Model file for the job. Use its own axes, mm. Face numbers are marked on the shaded views. A direction names the side the tool comes from. Coordinates: 2 decimals unless noted, no trailing zeros. Write each loop counter-clockwise with the first axis right and the second up, starting at its lowest first coordinate (ties: lowest second). Pieces come first, ordered by that corner, then holes. Notation, with made-up numbers: (76, 58.25) -> (98, 58.25) arc R31 ccw to (98, 85.25) -> close; hole circle Ø10 at (-12, 41). An arc over 180 degrees is marked (long way). Answer as a JSON object with one key per item and string values. Group by question number.
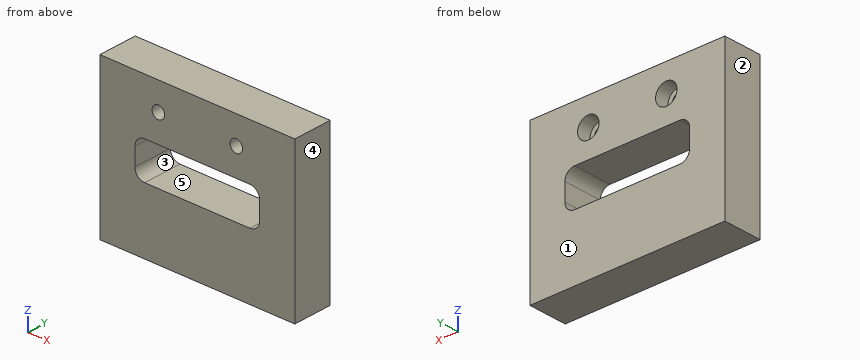
from build123d import *

# Parameters (mm, degrees)
SKETCH_1_W                = 100
SKETCH_1_H                = 80
SKETCH_1_W_2              = 64
SKETCH_1_H_2              = 19
EXTRUDE_1_DEPTH           = 20
FILLET_1_R                = 5
HOLE_WIZARD_1_D           = 6.4
HOLE_WIZARD_1_DEPTH       = 100
HOLE_WIZARD_1_CBORE_D     = 11
HOLE_WIZARD_1_CBORE_DEPTH = 7


with BuildPart() as part:
    # 草图1 → 凸台-拉伸1 (new body)
    with BuildSketch(Plane(origin=(0, 0, 0), x_dir=(1, 0, 0), z_dir=(0, 1, 0))):
        Rectangle(SKETCH_1_W, SKETCH_1_H)
        with Locations((0, -2.5)):
            Rectangle(SKETCH_1_W_2, SKETCH_1_H_2, mode=Mode.SUBTRACT)
    extrude(amount=EXTRUDE_1_DEPTH)

    # 圆角1
    fillet_1_edges = [part.edges().sort_by_distance(p)[0] for p in [
        (-32, 10, -7),
        (-32, 10, 12),
        (32, 10, 12),
        (32, 10, -7),
    ]]
    fillet(fillet_1_edges, radius=FILLET_1_R)

    # 孔1
    with Locations(Plane(origin=(0, 20, 0), x_dir=(1, 0, 0), z_dir=(0, 1, 0))):
        with Locations((20, -26), (-20, -26)):
            CounterBoreHole(HOLE_WIZARD_1_D / 2, HOLE_WIZARD_1_CBORE_D / 2, HOLE_WIZARD_1_CBORE_DEPTH, depth=HOLE_WIZARD_1_DEPTH)


solid = part.part
(1) Pull direction X, two halves, no side cores. Call the marked faces 1, 2 and 3: released by +X, released by -X, zero draft, split by the parting line, or undercut.
(2) Pin check, flat tips, straight feed: pin 1 (4 mm diameter, centred on x = 20, z = 26, fed in from -Y); pin 2 (3.5 mm diameter, centred on x = 18, z = 23.5, fed in from +Y). Stop position of each tip, or through.
(3) Cut at D-D on z = 26. List the corners of the cut face in (x, y).
(4) Cut at C-C on y = 9. List the corners of the cut face in (x, z).
(5) Cut at B-B on x = 20. List the corners of the cut face in (y, z).
(6) Cut at A-A on z = 10. List the corners of the cut face in (x, y).
(7) 3-axis set-ups, long thin cutter, end or side, ignore diameter. For the marked faces 4 and 5: which of +Z, -Z, +X, -X, +Y, -Y reach the whole face in a straight line?
(8) Wall check: probe 1 along Z at (x, y) = (-20, 6); probe 2 along X at (y, z) = (15.5, 26); probe 3 along X at (y, z) = (3.25, 26). Give the ranges that are in metal, low to high.
Results found:
{
 "1": {"face 1": "zero draft", "face 2": "released by -X", "face 3": "undercut"},
 "2": {"pin 1": "passes through", "pin 2": "stops at y = 13"},
 "3": {"outline": "(-50, 0) -> (-23.2, 0) -> (-23.2, 13) -> (-25.5, 13) -> (-25.5, 20) -> (-50, 20) -> close; (-16.8, 0) -> (16.8, 0) -> (16.8, 13) -> (14.5, 13) -> (14.5, 20) -> (-14.5, 20) -> (-14.5, 13) -> (-16.8, 13) -> close; (23.2, 0) -> (50, 0) -> (50, 20) -> (25.5, 20) -> (25.5, 13) -> (23.2, 13) -> close"},
 "4": {"outline": "(-50, -40) -> (50, -40) -> (50, 40) -> (-50, 40) -> close; hole (-32, -2) arc R5 ccw to (-27, -7) -> (27, -7) arc R5 ccw to (32, -2) -> (32, 7) arc R5 ccw to (27, 12) -> (-27, 12) arc R5 ccw to (-32, 7) -> close; hole circle Ø6.4 at (-20, 26); hole circle Ø6.4 at (20, 26)"},
 "5": {"outline": "(0, -40) -> (20, -40) -> (20, -7) -> (0, -7) -> close; (0, 12) -> (20, 12) -> (20, 20.5) -> (13, 20.5) -> (13, 22.8) -> (0, 22.8) -> close; (0, 29.2) -> (13, 29.2) -> (13, 31.5) -> (20, 31.5) -> (20, 40) -> (0, 40) -> close"},
 "6": {"outline": "(-50, 0) -> (-31, 0) -> (-31, 20) -> (-50, 20) -> close; (31, 0) -> (50, 0) -> (50, 20) -> (31, 20) -> close"},
 "7": {"face 4": "+Z, -Z, +X, +Y, -Y", "face 5": "+Y, -Y"},
 "8": {"probe 1": "z = -40 to -7, 12 to 22.8, 29.2 to 40", "probe 2": "x = -50 to -25.5, -14.5 to 14.5, 25.5 to 50", "probe 3": "x = -50 to -23.2, -16.8 to 16.8, 23.2 to 50"}
}
